Read the model definition and answer for the solid it produces. Units are mm, in the model's axes. Coordinates: 2 decimals unless noted, no trailing zeros. Loops run counter-clockwise (first coordinate to the right, second up) from the corner with the lowest first, then second, coordinate; pieces in that order, holes last. Notation, with made-up numbers: (52, 67) -> (59, 67) arc R29 cw to (59, 100) -> close; hole circle Ø2 at (80.5, 24.5). An arc over 180 degrees is marked (long way). Answer as a JSON object with one key per item and string values. Group by question number.
1) Section C-C, the plane y = 2 is taken. Give the vertices of the cut face in (x, z).
2) A flat-ended cylindrical pin translates along its axis: P1, Ø0.9, axis at x = 59, y = 1.5, coming from the +Z side. Find the tip coordinate at first contact, or state that the pin passes through.
3) Section D-D, the plane x = 64.5 is taken. Give the vertices of the cut face in (y, z), plus the area to 3 significant figures.
4) Section B-B, the plane z = -47.9 is taken. Count the separate pieces of the cut face and the enclosed holes in it, plus the area to 3 significant figures.
5) Section A-A, the plane x = 86.5 is taken. Give the vertices of the cut face in (y, z).
6) Consider probe 1 along Y at (x, z) = (53.5, -47.8); probe 2 along Y at (x, z) = (67.5, -44.65); probe 3 along Y at (x, z) = (71, -47.65). Determine where each line is inside the solid, lowest interval first. Write a range as [from, to].
from build123d import *

# Parameters (mm, degrees)
SKETCH1_W           = 100
SKETCH1_H           = 50
BOSS_EXTRUDE1_DEPTH = 6
SKETCH2_W           = 10
SKETCH2_H           = 3
CUT_EXTRUDE1_DEPTH  = 101
SKETCH3_W           = 6
SKETCH3_H           = 34
BOSS_EXTRUDE2_DEPTH = 100
SKETCH4_W           = 2
SKETCH4_H           = 5
CUT_EXTRUDE2_DEPTH  = 101
SKETCH5_W           = 7.857142857
SKETCH5_H           = 12.5
CUT_EXTRUDE3_DEPTH  = 5.7
CUT_EXTRUDE4_DEPTH  = 5.5
CUT_EXTRUDE5_DEPTH  = 101.0000001


with BuildPart() as part:
    # Sketch1 → Boss-Extrude1 (new body)
    with BuildSketch(Plane(origin=(0, 0, 0), x_dir=(1, 0, 0), z_dir=(0, 1, 0))):
        with Locations((50, 25)):
            Rectangle(SKETCH1_W, SKETCH1_H)
    extrude(amount=BOSS_EXTRUDE1_DEPTH)

    # Sketch2 → Cut-Extrude1 (cut, through all)
    with BuildSketch(Plane(origin=(100, 0, 0), x_dir=(0, 0, -1), z_dir=(1, 0, 0))):
        with Locations((5, 1.5)):
            Rectangle(SKETCH2_W, SKETCH2_H)
    extrude(amount=-CUT_EXTRUDE1_DEPTH, mode=Mode.SUBTRACT)

    # Sketch3 → Boss-Extrude2 (add)
    with BuildSketch(Plane(origin=(100, 0, 0), x_dir=(0, 0, -1), z_dir=(1, 0, 0))):
        with Locations((47, 17)):
            Rectangle(SKETCH3_W, SKETCH3_H)
    extrude(amount=-BOSS_EXTRUDE2_DEPTH)

    # Sketch4 → Cut-Extrude2 (cut, through all)
    with BuildSketch(Plane.ZY):
        with Locations((-45, 31.5)):
            Rectangle(SKETCH4_W, SKETCH4_H)
    extrude(amount=-CUT_EXTRUDE2_DEPTH, mode=Mode.SUBTRACT)

    # Sketch5 → Cut-Extrude3 (cut)
    with BuildSketch(Plane(origin=(0, 0, -44), x_dir=(-1, 0, 0), z_dir=(0, 0, -1))):
        with BuildLine():
            Line((-45.088169643, 17.571428571), (-45.439732143, 17.454241071))
            Line((-45.439732143, 17.454241071), (-48.056919643, 14.901227679))
            Line((-48.056919643, 14.901227679), (-48.098772321, 14.76171875))
            Line((-48.098772321, 14.76171875), (-48.107142857, 12.309151786))
            Line((-48.107142857, 12.309151786), (-48.059709821, 12.0859375))
            Line((-48.059709821, 12.0859375), (-45.609933036, 9.619419643))
            ThreePointArc((-45.609933036, 9.619419643), (-45.303061085, 9.424580045), (-44.945870536, 9.357142857))
            Line((-44.945870536, 9.357142857), (-38.319196429, 9.376674107))
            ThreePointArc((-38.319196429, 9.376674107), (-37.810119286, 9.488456034), (-37.392857143, 9.80078125))
            Line((-37.392857143, 9.80078125), (-37.392857143, 23.740513393))
            ThreePointArc((-37.392857143, 23.740513393), (-38.102358714, 23.844903984), (-38.818638393, 23.880022321))
            Line((-38.818638393, 23.880022321), (-38.821428571, 17.571428571))
            Line((-38.821428571, 17.571428571), (-40.116071429, 17.571428571))
            Line((-40.116071429, 17.571428571), (-46.991071429, 24.259486607))
            ThreePointArc((-46.991071429, 24.259486607), (-47.787451466, 24.334800239), (-48.031808036, 23.573102679))
            Line((-48.031808036, 23.573102679), (-41.681361607, 17.571428571))
            Line((-41.681361607, 17.571428571), (-45.088169643, 17.571428571))
        make_face()
        Polygon((-46.678571429, 12.557477679), (-44.725446429, 10.607142857), (-38.821428571, 10.607142857), (-38.821428571, 16.321428571), (-44.708705357, 16.321428571), (-46.678571429, 14.354352679), align=None, mode=Mode.SUBTRACT)
        with BuildLine():
            Line((-17.038504464, 9.619419643), (-19.48828125, 12.0859375))
            Line((-19.48828125, 12.0859375), (-19.535714286, 12.309151786))
            Line((-19.535714286, 12.309151786), (-19.52734375, 14.758928571))
            Line((-19.52734375, 14.758928571), (-19.485491071, 14.904017857))
            Line((-19.485491071, 14.904017857), (-16.896205357, 17.454241071))
            Line((-16.896205357, 17.454241071), (-16.555803571, 17.571428571))
            Line((-16.555803571, 17.571428571), (-10.25, 17.571428571))
            Line((-10.25, 17.571428571), (-10.244419643, 23.868861607))
            ThreePointArc((-10.244419643, 23.868861607), (-9.462763686, 24.582553037), (-8.821428571, 23.740513393))
            Line((-8.821428571, 23.740513393), (-8.821428571, 9.80078125))
            ThreePointArc((-8.821428571, 9.80078125), (-9.238690714, 9.488456034), (-9.747767857, 9.376674107))
            Line((-9.747767857, 9.376674107), (-16.374441964, 9.357142857))
            ThreePointArc((-16.374441964, 9.357142857), (-16.731632514, 9.424580045), (-17.038504464, 9.619419643))
        make_face()
        Polygon((-18.107142857, 12.563058036), (-16.154017857, 10.607142857), (-10.25, 10.607142857), (-10.25, 16.321428571), (-16.137276786, 16.321428571), (-18.107142857, 14.368303571), align=None, mode=Mode.SUBTRACT)
        with BuildLine():
            Line((-33.821428571, 10.1328125), (-33.815848214, 23.880022321))
            ThreePointArc((-33.815848214, 23.880022321), (-33.601713039, 24.293327013), (-33.140625, 24.357142857))
            Line((-33.140625, 24.357142857), (-23.508928571, 24.357142857))
            ThreePointArc((-23.508928571, 24.357142857), (-23.212822653, 23.985866281), (-23.107142857, 23.522879464))
            Line((-23.107142857, 23.522879464), (-23.107142857, 9.78125))
            ThreePointArc((-23.107142857, 9.78125), (-23.280423047, 9.477022359), (-23.609375, 9.357142857))
            Line((-23.609375, 9.357142857), (-33.235491071, 9.379464286))
            ThreePointArc((-33.235491071, 9.379464286), (-33.657785084, 9.655552078), (-33.821428571, 10.1328125))
        make_face()
        with Locations((-28.464285715, 16.857142857)):
            Rectangle(SKETCH5_W, SKETCH5_H, mode=Mode.SUBTRACT)
        with BuildLine():
            Line((-62.392857143, 10.1328125), (-62.387276786, 23.880022321))
            ThreePointArc((-62.387276786, 23.880022321), (-62.17314161, 24.293327013), (-61.712053571, 24.357142857))
            Line((-61.712053571, 24.357142857), (-52.080357143, 24.357142857))
            ThreePointArc((-52.080357143, 24.357142857), (-51.784251224, 23.985866281), (-51.678571429, 23.522879464))
            Line((-51.678571429, 23.522879464), (-51.678571429, 9.78125))
            ThreePointArc((-51.678571429, 9.78125), (-51.851851619, 9.477022359), (-52.180803571, 9.357142857))
            Line((-52.180803571, 9.357142857), (-61.806919643, 9.379464286))
            ThreePointArc((-61.806919643, 9.379464286), (-62.283572717, 9.613272807), (-62.392857143, 10.1328125))
        make_face()
        with Locations((-57.035714286, 16.857142857)):
            Rectangle(SKETCH5_W, SKETCH5_H, mode=Mode.SUBTRACT)
        with BuildLine():
            Line((-76.516741071, 10.224888393), (-69.834263393, 16.890625))
            Line((-69.834263393, 16.890625), (-76.508370536, 23.564732143))
            ThreePointArc((-76.508370536, 23.564732143), (-76.263865977, 24.33823157), (-75.456473214, 24.259486607))
            Line((-75.456473214, 24.259486607), (-68.670758929, 17.571428571))
            Line((-68.670758929, 17.571428571), (-67.392857143, 17.571428571))
            Line((-67.392857143, 17.571428571), (-67.390066964, 23.880022321))
            ThreePointArc((-67.390066964, 23.880022321), (-66.613914042, 24.456808533), (-65.964285714, 23.740513393))
            Line((-65.964285714, 23.740513393), (-65.964285714, 9.789620536))
            ThreePointArc((-65.964285714, 9.789620536), (-66.815504738, 9.403127861), (-67.392857143, 10.138392857))
            Line((-67.392857143, 10.138392857), (-67.392857143, 16.321428571))
            Line((-67.392857143, 16.321428571), (-68.66796875, 16.321428571))
            Line((-68.66796875, 16.321428571), (-75.489955357, 9.465959821))
            ThreePointArc((-75.489955357, 9.465959821), (-76.031889018, 9.806810078), (-76.516741071, 10.224888393))
        make_face()
        with BuildLine():
            Line((-81.678571429, 10.130022321), (-81.678571429, 21.2265625))
            Line((-81.678571429, 21.2265625), (-83.5703125, 23.107142857))
            Line((-83.5703125, 23.107142857), (-87.585379464, 23.107142857))
            Line((-87.585379464, 23.107142857), (-89.535714286, 21.151227679))
            Line((-89.535714286, 21.151227679), (-89.535714286, 9.770089286))
            ThreePointArc((-89.535714286, 9.770089286), (-90.273009404, 9.862916097), (-90.964285714, 10.135602679))
            Line((-90.964285714, 10.135602679), (-90.883370536, 21.751116071))
            Line((-90.883370536, 21.751116071), (-88.2578125, 24.320870536))
            Line((-88.2578125, 24.320870536), (-87.872767857, 24.357142857))
            Line((-87.872767857, 24.357142857), (-82.970424107, 24.357142857))
            Line((-82.970424107, 24.357142857), (-82.7890625, 24.234375))
            Line((-82.7890625, 24.234375), (-80.303013393, 21.742745536))
            Line((-80.303013393, 21.742745536), (-80.25, 21.48046875))
            Line((-80.25, 21.48046875), (-80.25, 9.78125))
            ThreePointArc((-80.25, 9.78125), (-80.985264996, 9.869705022), (-81.678571429, 10.130022321))
        make_face()
    extrude(amount=CUT_EXTRUDE3_DEPTH, mode=Mode.SUBTRACT)

    # Sketch8 → Cut-Extrude4 (cut)
    with BuildSketch(Plane(origin=(0, 6, 0), x_dir=(1, 0, 0), z_dir=(0, 1, 0))):
        with BuildLine():
            Line((7.011617647, 30.077205882), (8.955082743, 27.33260299))
            add(Edge.make_bspline(
                [(8.955082743, 27.33260299), (9.12959235, 26.730722395), (8.207708735, 26.573406529), (7.899470003, 26.933823529)],
                knots=[0, 0, 0, 0, 1, 1, 1, 1], degree=3))
            add(Edge.make_bspline(
                [(7.899470003, 26.933823529), (6.967481131, 27.995956124), (6.173874947, 29.162344961)],
                knots=[0, 0, 0, 1, 1, 1], degree=2))
            add(Edge.make_bspline(
                [(6.173874947, 29.162344961), (5.827065663, 29.66494419), (6.530628947, 30.242627585), (7.011617647, 30.077205882)],
                knots=[0, 0, 0, 0, 1, 1, 1, 1], degree=3))
        make_face()
        with BuildLine():
            Line((8.476184036, 31.013434386), (10.320441176, 28.506054806))
            add(Edge.make_bspline(
                [(10.320441176, 28.506054806), (10.75287522, 28.022402696), (9.844480118, 27.32594185), (9.464423283, 27.806698869)],
                knots=[0, 0, 0, 0, 1, 1, 1, 1], degree=3))
            add(Edge.make_bspline(
                [(7.548449232, 30.408088235), (8.369245022, 29.00368602), (9.464423283, 27.806698869)],
                knots=[0, 0, 0, 1, 1, 1], degree=2))
            add(Edge.make_bspline(
                [(7.548449232, 30.408088235), (7.420862108, 30.780822958), (7.657281624, 31.572935659), (8.169705882, 31.400735294)],
                knots=[0, 0, 0, 0, 1, 1, 1, 1], degree=3))
            add(Edge.make_bspline(
                [(8.169705882, 31.400735294), (8.365163665, 31.240936083), (8.476184036, 31.013434386)],
                knots=[0, 0, 0, 1, 1, 1], degree=2))
        make_face()
        Polygon((10.816764706, 31.400735294), (10.155, 32.724264706), (9.327794118, 32.393382353), (9.162352941, 31.235294118), (9.824117647, 30.408088235), align=None)
        with BuildLine():
            Line((12.802058824, 32.227941176), (11.643970588, 33.716911765))
            add(Edge.make_bspline(
                [(11.643970588, 33.716911765), (10.801410064, 33.411012177), (11.092331374, 32.550744981)],
                knots=[0, 0, 0, 1, 1, 1], degree=2))
            Line((11.092331374, 32.550744981), (11.643970588, 31.731617647))
            Line((11.643970588, 31.731617647), (12.802058824, 32.227941176))
        make_face()
        with BuildLine():
            Line((13.193009945, 29.973529412), (13.854774651, 28.815441176))
            Line((13.854774651, 28.815441176), (8.560657004, 26.333823529))
            Line((8.560657004, 26.333823529), (7.402568768, 26.830147059))
            Line((7.402568768, 26.830147059), (9.056980533, 19.881617647))
            Line((9.056980533, 19.881617647), (13.689333474, 20.047058824))
            add(Edge.make_bspline(
                [(13.689333474, 20.047058824), (12.450227116, 27.171920383), (13.777231511, 23.836713066), (15.840068768, 28.65)],
                knots=[0, 0, 0, 0, 1, 1, 1, 1], degree=3))
            Line((15.840068768, 28.65), (13.854774651, 31.627941176))
            Line((13.854774651, 31.627941176), (10.711392298, 30.138970588))
            Line((10.711392298, 30.138970588), (12.365804063, 29.477205882))
            Line((12.365804063, 29.477205882), (13.193009945, 29.973529412))
        make_face()
        Polygon((31.240068768, 25.85), (31.240068768, 28.65), (28.440068768, 28.65), (28.440068768, 31.45), (25.640068768, 31.45), (25.640068768, 28.65), (22.840068768, 28.65), (22.840068768, 25.85), (25.640068768, 25.85), (25.640068768, 23.05), (28.440068768, 23.05), (28.440068768, 25.85), align=None)
        Polygon((52.041417767, 30.75), (42.541417767, 30.75), (42.541417767, 33.75), (37.990068768, 27.25), (42.541417767, 20.75), (42.541417767, 23.75), (52.041417767, 23.75), align=None)
        Polygon((60.419322104, 21.339322104), (59.041417767, 29.153805922), (61.16273811, 27.032485579), (67.880252532, 33.75), (72.83, 28.800252532), (66.112485579, 22.08273811), (68.233805922, 19.961417767), align=None)
        Polygon((90.03, 33.75), (90.03, 24.25), (93.03, 24.25), (86.476783646, 19.661388509), (80.03, 24.25), (83.03, 24.25), (83.03, 33.75), align=None)
    extrude(amount=-CUT_EXTRUDE4_DEPTH, mode=Mode.SUBTRACT)

    # Sketch9 → Cut-Extrude5 (cut, through all)
    with BuildSketch(Plane.ZY):
        Polygon((0, 6), (-44, 6), (-44, 3), (-47, 3), (-47, 0), (-44, 0), (0, 0), align=None)
    extrude(amount=-CUT_EXTRUDE5_DEPTH, mode=Mode.SUBTRACT)


solid = part.part
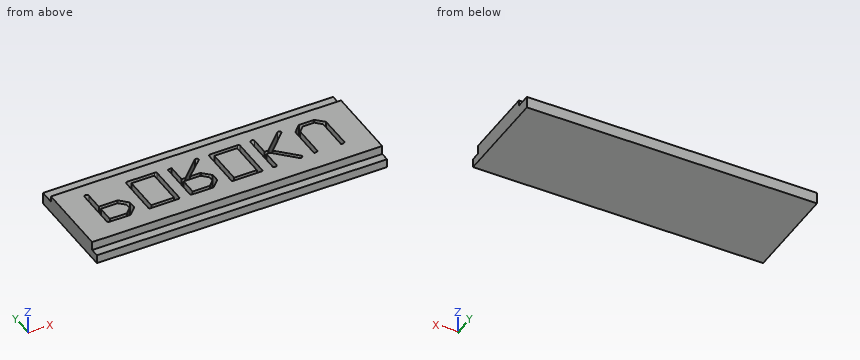
Determined:
{
 "1": {"outline": "(0, -50) -> (100, -50) -> (100, -47) -> (0, -47) -> close"},
 "2": {"P1": "z = -47"},
 "3": {"outline": "(0, -50) -> (34, -50) -> (34, -46) -> (29, -46) -> (29, -44) -> (3, -44) -> (3, -47) -> (0, -47) -> close", "area": "185 mm²"},
 "4": {"separate pieces": "5", "enclosed holes": "6", "area": "3,070 mm²"},
 "5": {"outline": "(0, -50) -> (34, -50) -> (34, -46) -> (29, -46) -> (29, -44) -> (24.36, -44) -> (24.36, -49.7) -> (23.11, -49.7) -> (23.11, -44) -> (3, -44) -> (3, -47) -> (0, -47) -> close"},
 "6": {"probe 1": "[0, 9.36], [10.61, 23.11], [24.36, 34]", "probe 2": "[3, 16.32], [17.57, 29]", "probe 3": "[0, 13.98], [15.73, 18.06], [19.87, 34]"}
}
